from build123d import *

# Parameters (mm, degrees)
SKETCH_2_W      = 0.7
SKETCH_2_H      = 4.413249275
SKETCH_3_W      = 6
SKETCH_3_H      = 5.5
EXTRUDE_1_DEPTH = 14
SKETCH_4_R      = 0.35
EXTRUDE_2_DEPTH = 4.3


with BuildPart() as part:
    # 草图1 → 旋转1 (revolve)
    with BuildSketch(Plane.XY, mode=Mode.PRIVATE) as revolve_1_sk:
        Polygon((0, 10), (1, 10), (1, 5.95), (24, 5.95), (24, 10), (25, 10), (25, 5.325), (0, 5.325), align=None)
    revolve(revolve_1_sk.sketch.rotate(Axis((15.438516229, 0, 0), (-1, 0, 0)), 90), axis=Axis((15.438516229, 0, 0), (-1, 0, 0)))

    # 草图2 → 旋转2 (revolve)
    with BuildSketch(Plane.XY, mode=Mode.PRIVATE) as revolve_2_sk:
        with Locations((7.75, 7.589473804)):
            Rectangle(SKETCH_2_W, SKETCH_2_H)
        with Locations((10.55, 7.589473804)):
            Rectangle(SKETCH_2_W, SKETCH_2_H)
        with Locations((13.35, 7.589473804)):
            Rectangle(SKETCH_2_W, SKETCH_2_H)
        with Locations((16.05, 7.589473804)):
            Rectangle(SKETCH_2_W, SKETCH_2_H)
        with Locations((18.75, 7.589473804)):
            Rectangle(SKETCH_2_W, SKETCH_2_H)
        with Locations((21.5, 7.589473804)):
            Rectangle(SKETCH_2_W, SKETCH_2_H)
    revolve(revolve_2_sk.sketch.rotate(Axis((-4.318730042, 0, 0), (1, 0, 0)), 270), axis=Axis((-4.318730042, 0, 0), (1, 0, 0)))

    # 草图3 → 凸台-拉伸1 (add, symmetric)
    with BuildSketch(Plane.XY):
        with Locations((-2, -8.075)):
            Rectangle(SKETCH_3_W, SKETCH_3_H)
        with Locations((27, -8.075)):
            Rectangle(SKETCH_3_W, SKETCH_3_H)
    extrude(amount=EXTRUDE_1_DEPTH, both=True)

    # 草图4 → 凸台-拉伸2 (add)
    with BuildSketch(Plane.XZ.offset(10.825)):
        with Locations(Location((-0.5, 12.5, 0), (0, 0, 180))):
            Circle(SKETCH_4_R)
        with Locations(Location((-0.5, 7.5, 0), (0, 0, 180))):
            Circle(SKETCH_4_R)
        with Locations(Location((-0.5, 2.5, 0), (0, 0, 180))):
            Circle(SKETCH_4_R)
        with Locations(Location((-0.5, -2.5, 0), (0, 0, 180))):
            Circle(SKETCH_4_R)
        with Locations(Location((-0.5, -7.5, 0), (0, 0, 180))):
            Circle(SKETCH_4_R)
        with Locations(Location((-0.5, -12.5, 0), (0, 0, 180))):
            Circle(SKETCH_4_R)
        with Locations(Location((25.5, -12.5, 0), (0, 0, 90))):
            Circle(SKETCH_4_R)
        with Locations(Location((25.5, -7.5, 0), (0, 0, 90))):
            Circle(SKETCH_4_R)
        with Locations(Location((25.5, -2.5, 0), (0, 0, 90))):
            Circle(SKETCH_4_R)
        with Locations(Location((25.5, 2.5, 0), (0, 0, 90))):
            Circle(SKETCH_4_R)
        with Locations(Location((25.5, 7.5, 0), (0, 0, 90))):
            Circle(SKETCH_4_R)
        with Locations(Location((25.5, 12.5, 0), (0, 0, 90))):
            Circle(SKETCH_4_R)
    extrude(amount=EXTRUDE_2_DEPTH)


solid = part.part
Here's how the part is built. I have some questions about the finished solid (model axes, mm). A direction names the side the tool comes from. Coordinates: 2 decimals unless noted, no trailing zeros. Write each loop counter-clockwise with the first axis right and the second up, starting at its lowest first coordinate (ties: lowest second). Pieces come first, ordered by that corner, then holes.
Item 1: On a 3-axis mill with a long thin cutter (end or side, diameter ignored), from which of +Z, -Z, +X, -X, +Y, -Y can I reach the whole of each face in a straight line? I mean faces 1 (the cylindrical face through (7.75, 8.26, -5.27)), 2 (the flat face through (-2, -8, 14)), 3 (the flat face through (25, 6, 0)). Say none if no direction works.
Item 2: I want a section at A-A on y = -12. Count the separate pieces of the cut face and the enclosed holes in it, and give its area (3 significant figures).
Item 3: Will these pins go through, and if not, where does the flat tip stop? pin 1 (1 mm diameter, centred on y = -4, z = -9, fed in from +X); pin 2 (5 mm diameter, centred on y = -12, z = 2.5, fed in from -X); pin 3 (1.5 mm diameter, centred on x = 6, y = -2.5, fed in from -Z); pin 4 (4 mm diameter, centred on x = 25.5, y = 5.5, fed in from +Z).
Item 4: I want a section at C-C on x = 24.5. Write out the boundary of the cut face in (y, z) (3 decimals).
Item 5: If I drill on line 1 (Y direction, x = 19.75, z = 0) (3 decimals); line 2 (Y direction, x = 10.25, z = 0) (3 decimals); line 3 (X direction, y = -10.5, z = -8.25), over which ranges is the centre line in solid material (lowest first)?
Findings below:
1. face 1: none
1. face 2: +Z, +X, -X, +Y, -Y
1. face 3: +Z, -Z, +X, +Y
2. separate pieces: 12
2. enclosed holes: 0
2. area: 4.62 mm2
3. pin 1: stops at x = 25
3. pin 2: stops at x = -5
3. pin 3: stops at z = -5.69
3. pin 4: stops at z = 9.34
4. outline: (-10.825, -14) - (-5.325, -14) - (-5.325, -8.464) arc R10 ccw (long way) to (-5.325, 8.464) - (-5.325, 14) - (-10.825, 14) - close; hole circle Ø10.65 at (0, 0)
5. line 1: y = -5.95 to -5.325, 5.325 to 5.95
5. line 2: y = -9.796 to -5.325, 5.325 to 9.796
5. line 3: x = -5 to 1, 24 to 30
